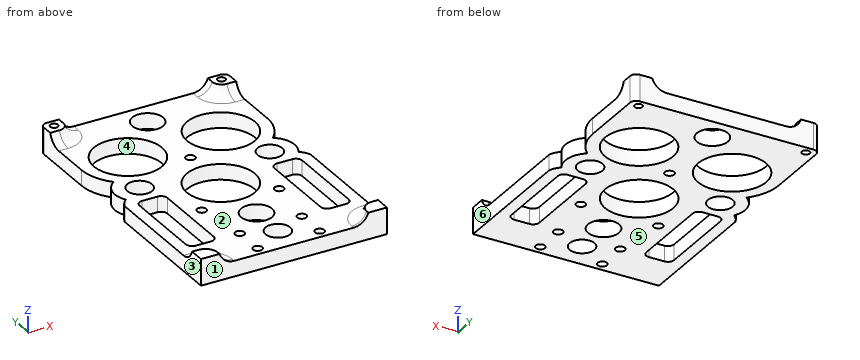
from build123d import *

# Parameters (mm, degrees)
SKETCH1_W            = 60
SKETCH1_H            = 90
BOSS_EXTRUDE1_DEPTH  = 5
SKETCH2_W            = 9
SKETCH2_H            = 30
CUT_EXTRUDE1_DEPTH   = 55.313902456
FILLET1_R            = 2
BOSS_EXTRUDE2_DEPTH  = 3.5
FILLET2_R            = 5
FILLET2_OF_MIRROR1_R = 5
BOSS_EXTRUDE3_DEPTH  = 3.5
SKETCH5_R            = 1.25
CUT_EXTRUDE2_DEPTH   = 55.747146044
FILLET3_R            = 5
FILLET3_OF_MIRROR4_R = 5
FILLET4_R            = 2
SKETCH6_R            = 1.5
CUT_EXTRUDE3_DEPTH   = 55.747146044
SKETCH7_R            = 11
SKETCH7_R_2          = 5
SKETCH7_R_3          = 4
CUT_EXTRUDE4_DEPTH   = 55.313902456


with BuildPart() as part:
    # Sketch1 → Boss-Extrude1 (new body)
    with BuildSketch(Plane.XY):
        Rectangle(SKETCH1_W, SKETCH1_H)
    extrude(amount=BOSS_EXTRUDE1_DEPTH)

    # Sketch2 → Cut-Extrude1 (cut, through all)
    with BuildSketch(Plane(origin=(0, 0, 0), x_dir=(-1, 0, 0), z_dir=(0, 0, -1))):
        with Locations((-21.75, -17)):
            Rectangle(SKETCH2_W, SKETCH2_H)
        with Locations((21.75, -17)):
            Rectangle(SKETCH2_W, SKETCH2_H)
    extrude(amount=-CUT_EXTRUDE1_DEPTH, mode=Mode.SUBTRACT)

    # Fillet1
    fillet1_edges = [part.edges().sort_by_distance(p)[0] for p in [
        (26.25, -32, 2.5),
        (26.25, -2, 2.5),
        (17.25, -2, 2.5),
        (17.25, -32, 2.5),
        (-17.25, -32, 2.5),
        (-17.25, -2, 2.5),
        (-26.25, -2, 2.5),
        (-26.25, -32, 2.5),
    ]]
    fillet(fillet1_edges, radius=FILLET1_R)

    # Sketch3 → Boss-Extrude2 (add)
    with BuildSketch(Plane.XY.offset(5)):
        with BuildLine():
            Line((28, -40), (30, -40))
            Line((30, -40), (30, -45))
            Line((30, -45), (24, -45))
            Line((24, -45), (24, -44))
            ThreePointArc((24, -44), (25.171572875, -41.171572875), (28, -40))
        make_face()
    boss_extrude2 = extrude(amount=BOSS_EXTRUDE2_DEPTH)

    # Fillet2
    # the kernel refuses this fillet: 5 mm, written as the material it adds along each edge
    with BuildSketch(Plane(origin=(28, -40, 5), x_dir=(0, 1, 0), z_dir=(1, 0, 0))) as fillet2_piece_1:
        with BuildLine():
            CenterArc((4.769696007, 5), FILLET2_R, 197.457603124, 72.542396876)
            Line((0, 3.5), (-0.09539392, 3.47))
            ThreePointArc((-0.09539392, 3.47), (-0.1, 1.75), (-0.1, 0))
            Line((-0.1, 0), (0, -0.1))
            Line((0, -0.1), (4.769696007, -0.1))
            Line((4.769696007, -0.1), (4.769696007, 0))
        make_face()
    extrude(amount=2)
    with BuildSketch(Plane(origin=(24, -45, 5), x_dir=(-1, 0, 0), z_dir=(0, 1, 0))) as fillet2_piece_2:
        with BuildLine():
            CenterArc((4.769696007, 5), FILLET2_R, 197.457603124, 72.542396876)
            Line((0, 3.5), (-0.09539392, 3.47))
            ThreePointArc((-0.09539392, 3.47), (-0.1, 1.75), (-0.1, 0))
            Line((-0.1, 0), (0, -0.1))
            Line((0, -0.1), (4.769696007, -0.1))
            Line((4.769696007, -0.1), (4.769696007, 0))
        make_face()
    extrude(amount=1)
    with BuildSketch(Plane(origin=(28, -44, 5), x_dir=(-1, 0, 0), z_dir=(0, -1, 0))) as fillet2_piece_3:
        with BuildLine():
            CenterArc((8.769696007, -5), FILLET2_R, 90, 72.542396876)
            Line((4, -3.5), (3.90460608, -3.47))
            ThreePointArc((3.90460608, -3.47), (3.9, -1.75), (3.9, 0))
            Line((3.9, 0), (4, 0.1))
            Line((4, 0.1), (8.769696007, 0.1))
            Line((8.769696007, 0.1), (8.769696007, 0))
        make_face()
    revolve(axis=Axis((28, -44, 5), (0, 0, -1)), revolution_arc=90)

    # Mirror1: Boss-Extrude2 across plane
    add(boss_extrude2.mirror(Plane(origin=(0, 0, 0), x_dir=(0, 0, 1), z_dir=(1, 0, 0))))

    # Fillet2 of Mirror1
    # the kernel refuses this fillet: 5 mm, written as the material it adds along each edge
    with BuildSketch(Plane(origin=(-28, -40, 5), x_dir=(0, 0, 1), z_dir=(-1, 0, 0))) as fillet2_of_mirror1_piece_1:
        with BuildLine():
            CenterArc((5, 4.769696007), FILLET2_OF_MIRROR1_R, 180, 72.542396876)
            Line((0, 4.769696007), (-0.1, 4.769696007))
            Line((-0.1, 4.769696007), (-0.1, 0))
            Line((-0.1, 0), (0, -0.1))
            ThreePointArc((0, -0.1), (1.75, -0.1), (3.47, -0.09539392))
            Line((3.47, -0.09539392), (3.5, 0))
        make_face()
    extrude(amount=2)
    with BuildSketch(Plane(origin=(-24, -45, 5), x_dir=(0, 0, 1), z_dir=(0, 1, 0))) as fillet2_of_mirror1_piece_2:
        with BuildLine():
            CenterArc((5, 4.769696007), FILLET2_OF_MIRROR1_R, 180, 72.542396876)
            Line((0, 4.769696007), (-0.1, 4.769696007))
            Line((-0.1, 4.769696007), (-0.1, 0))
            Line((-0.1, 0), (0, -0.1))
            ThreePointArc((0, -0.1), (1.75, -0.1), (3.47, -0.09539392))
            Line((3.47, -0.09539392), (3.5, 0))
        make_face()
    extrude(amount=1)
    with BuildSketch(Plane(origin=(-28, -44, 5), x_dir=(1, 0, 0), z_dir=(0, -1, 0))) as fillet2_of_mirror1_piece_3:
        with BuildLine():
            CenterArc((8.769696007, 5), FILLET2_OF_MIRROR1_R, 197.457603124, 72.542396876)
            Line((8.769696007, 0), (8.769696007, -0.1))
            Line((8.769696007, -0.1), (4, -0.1))
            Line((4, -0.1), (3.9, 0))
            ThreePointArc((3.9, 0), (3.9, 1.75), (3.90460608, 3.47))
            Line((3.90460608, 3.47), (4, 3.5))
        make_face()
    revolve(axis=Axis((-28, -44, 5), (0, 0, 1)), revolution_arc=90)

    # Sketch4 → Boss-Extrude3 (add)
    with BuildSketch(Plane.XY.offset(5)):
        with BuildLine():
            Line((24, 45), (24, 42.5))
            ThreePointArc((24, 42.5), (24.878679656, 40.378679656), (27, 39.5))
            Line((27, 39.5), (30, 39.5))
            Line((30, 39.5), (30, 45))
            Line((30, 45), (24, 45))
        make_face()
    boss_extrude3 = extrude(amount=BOSS_EXTRUDE3_DEPTH)

    # Sketch5 → Cut-Extrude2 (cut, through all)
    with BuildSketch(Plane.XY.offset(8.5)):
        with Locations((27, 42.5)):
            Circle(SKETCH5_R)
    cut_extrude2 = extrude(amount=-CUT_EXTRUDE2_DEPTH, mode=Mode.SUBTRACT)

    # Fillet3
    # the kernel refuses this fillet: 5 mm, written as the material it adds along each edge
    with BuildSketch(Plane(origin=(24, 45, 5), x_dir=(-1, 0, 0), z_dir=(0, -1, 0))) as fillet3_piece_1:
        with BuildLine():
            CenterArc((4.769696007, -5), FILLET3_R, 90, 72.542396876)
            Line((0, -3.5), (-0.09539392, -3.47))
            ThreePointArc((-0.09539392, -3.47), (-0.1, -1.75), (-0.1, 0))
            Line((-0.1, 0), (0, 0.1))
            Line((0, 0.1), (4.769696007, 0.1))
            Line((4.769696007, 0.1), (4.769696007, 0))
        make_face()
    extrude(amount=2.5)
    with BuildSketch(Plane(origin=(27, 42.5, 5), x_dir=(-1, 0, 0), z_dir=(0, 1, 0))) as fillet3_piece_2:
        with BuildLine():
            CenterArc((7.769696007, 5), FILLET3_R, 197.457603124, 72.542396876)
            Line((3, 3.5), (2.90460608, 3.47))
            ThreePointArc((2.90460608, 3.47), (2.9, 1.75), (2.9, 0))
            Line((2.9, 0), (3, -0.1))
            Line((3, -0.1), (7.769696007, -0.1))
            Line((7.769696007, -0.1), (7.769696007, 0))
        make_face()
    revolve(axis=Axis((27, 42.5, 5), (0, 0, 1)), revolution_arc=90)
    with BuildSketch(Plane(origin=(27, 39.5, 5), x_dir=(0, -1, 0), z_dir=(1, 0, 0))) as fillet3_piece_3:
        with BuildLine():
            CenterArc((4.769696007, -5), FILLET3_R, 90, 72.542396876)
            Line((0, -3.5), (-0.09539392, -3.47))
            ThreePointArc((-0.09539392, -3.47), (-0.1, -1.75), (-0.1, 0))
            Line((-0.1, 0), (0, 0.1))
            Line((0, 0.1), (4.769696007, 0.1))
            Line((4.769696007, 0.1), (4.769696007, 0))
        make_face()
    extrude(amount=3)

    # Mirror4: Boss-Extrude3, Cut-Extrude2 across plane
    add(boss_extrude3.mirror(Plane(origin=(0, 0, 0), x_dir=(0, 0, 1), z_dir=(1, 0, 0))))
    add(cut_extrude2.mirror(Plane(origin=(0, 0, 0), x_dir=(0, 0, 1), z_dir=(1, 0, 0))), mode=Mode.SUBTRACT)

    # Fillet3 of Mirror4
    # the kernel refuses this fillet: 5 mm, written as the material it adds along each edge
    with BuildSketch(Plane(origin=(-24, 45, 5), x_dir=(1, 0, 0), z_dir=(0, -1, 0))) as fillet3_of_mirror4_piece_1:
        with BuildLine():
            CenterArc((4.769696007, 5), FILLET3_OF_MIRROR4_R, 197.457603124, 72.542396876)
            Line((0, 3.5), (-0.09539392, 3.47))
            ThreePointArc((-0.09539392, 3.47), (-0.1, 1.75), (-0.1, 0))
            Line((-0.1, 0), (0, -0.1))
            Line((0, -0.1), (4.769696007, -0.1))
            Line((4.769696007, -0.1), (4.769696007, 0))
        make_face()
    extrude(amount=2.5)
    with BuildSketch(Plane(origin=(-27, 42.5, 5), x_dir=(1, 0, 0), z_dir=(0, 1, 0))) as fillet3_of_mirror4_piece_2:
        with BuildLine():
            CenterArc((7.769696007, -5), FILLET3_OF_MIRROR4_R, 90, 72.542396876)
            Line((3, -3.5), (2.90460608, -3.47))
            ThreePointArc((2.90460608, -3.47), (2.9, -1.75), (2.9, 0))
            Line((2.9, 0), (3, 0.1))
            Line((3, 0.1), (7.769696007, 0.1))
            Line((7.769696007, 0.1), (7.769696007, 0))
        make_face()
    revolve(axis=Axis((-27, 42.5, 5), (0, 0, -1)), revolution_arc=90)
    with BuildSketch(Plane(origin=(-27, 39.5, 5), x_dir=(0, -1, 0), z_dir=(-1, 0, 0))) as fillet3_of_mirror4_piece_3:
        with BuildLine():
            CenterArc((4.769696007, 5), FILLET3_OF_MIRROR4_R, 197.457603124, 72.542396876)
            Line((0, 3.5), (-0.09539392, 3.47))
            ThreePointArc((-0.09539392, 3.47), (-0.1, 1.75), (-0.1, 0))
            Line((-0.1, 0), (0, -0.1))
            Line((0, -0.1), (4.769696007, -0.1))
            Line((4.769696007, -0.1), (4.769696007, 0))
        make_face()
    extrude(amount=3)

    # Fillet4
    fillet4_edges = [part.edges().sort_by_distance(p)[0] for p in [
        (-30, 45, 4.25),
        (30, 45, 4.25),
    ]]
    fillet(fillet4_edges, radius=FILLET4_R)

    # Sketch6 → Cut-Extrude3 (cut, through all)
    with BuildSketch(Plane(origin=(0, 0, 0), x_dir=(-1, 0, 0), z_dir=(0, 0, -1))):
        with Locations((-10, -32)):
            Circle(SKETCH6_R)
        with Locations((-10, -42)):
            Circle(SKETCH6_R)
        with Locations((10, -42)):
            Circle(SKETCH6_R)
        with Locations((10, -32)):
            Circle(SKETCH6_R)
        with Locations((0, 13)):
            Circle(SKETCH6_R)
        with Locations((12.5, -15)):
            Circle(SKETCH6_R)
        with Locations((-12.5, -15)):
            Circle(SKETCH6_R)
    extrude(amount=-CUT_EXTRUDE3_DEPTH, mode=Mode.SUBTRACT)

    # Sketch7 → Cut-Extrude4 (cut, through all)
    with BuildSketch(Plane.XY.offset(5)):
        with Locations((-15, 22)):
            Circle(SKETCH7_R)
        with Locations((15, 22)):
            Circle(SKETCH7_R)
        with Locations((0, -4)):
            Circle(SKETCH7_R)
        with Locations((0, -24)):
            Circle(SKETCH7_R_2)
        with Locations((0, -36)):
            Circle(SKETCH7_R_3)
        with Locations((0, 37)):
            Circle(SKETCH7_R_2)
        with Locations((-21, 5)):
            Circle(SKETCH7_R_3)
        with Locations((21, 5)):
            Circle(SKETCH7_R_3)
        with BuildLine():
            Line((30, 22), (30, 5))
            Line((30, 5), (30, -2.28608635))
            ThreePointArc((30, -2.28608635), (29.162980054, -0.555783544), (27.82175868, 0.821051746))
            ThreePointArc((27.82175868, 0.821051746), (28.844928487, 6.567513007), (25.692059794, 11.479550516))
            ThreePointArc((25.692059794, 11.479550516), (28.881298515, 16.315850852), (30, 22))
        make_face()
        with BuildLine():
            Line((-30, 5), (-30, -2.28608635))
            ThreePointArc((-30, -2.28608635), (-29.162980054, -0.555783544), (-27.82175868, 0.821051746))
            ThreePointArc((-27.82175868, 0.821051746), (-28.844928487, 6.567513007), (-25.692059794, 11.479550516))
            ThreePointArc((-25.692059794, 11.479550516), (-28.881298515, 16.315850852), (-30, 22))
            Line((-30, 22), (-30, 5))
        make_face()
    extrude(amount=-CUT_EXTRUDE4_DEPTH, mode=Mode.SUBTRACT)


solid = part.part
The listing builds one solid part. Answer for the finished solid, in the listing's coordinates (mm). Face numbers are marked on the shaded views. A direction names the side the tool comes from. Coordinates: 2 decimals unless noted, no trailing zeros. Order: outer loops, then holes, each group sorted by start corner. A loop starts at its lowest first (then second) coordinate and runs counter-clockwise, first axis right, second up. Notation, with made-up numbers: M 53.5,29 L 71.5,29 A15 cw 71.5,41 Z; hole C 22,-19 d7. An arc over 180 degrees is marked long. Use CSV: the item, a comma, the result in double quotes.
Q1. Section D-D (x = 10) is taken. Determine the outline of the cut face in (y, z).
Here are the results:
outline,"M -45,0 L -43.5,0 L -43.5,5 L -45,5 Z; M -40.5,0 L -33.5,0 L -33.5,5 L -40.5,5 Z; M -30.5,0 L -8.58,0 L -8.58,5 L -30.5,5 Z; M 0.58,0 L 12.2,0 L 12.2,5 L 0.58,5 Z; M 31.8,0 L 45,0 L 45,5 L 31.8,5 Z"
Q2. Determine the mould class of the marked faces 3, 4, 5 and 6 for opening direction X: pulls with the +X half, pulls with the -X half, needs draft (parallel to the pull), parting line crosses it, or undercut.
Here are the results:
face 3,"pulls with the -X half"
face 4,"undercut"
face 5,"needs draft"
face 6,"pulls with the +X half"
Q3. A tool of negligible diameter and unlimited length cuts with its end or side. For the marked faces 1 and 2, from which of +Z, -Z, +X, -X, +Y, -Y can it reach the whole face along a straight path? Write none if from no direction.
Here are the results:
face 1,"+Z, -Z, +X, -X, -Y"
face 2,"+Z"
Q4. Straight lines are drawn through the part: L1, parallel to Y at x = 0, z = 1.1; L2, parallel to Y at x = 7.5, z = 1.5; L3, parallel to X at y = 25.5, z = 1.5. For each, find the intervals that lie inside material, in ascending order.
Here are the results:
L1,"-45 to -40, -32 to -29, -19 to -15, 7 to 11.5, 14.5 to 32, 42 to 45"
L2,"-45 to -12.05, 4.05 to 13.95, 30.05 to 45"
L3,"-30 to -25.43, -4.57 to 4.57, 25.43 to 30"
Q5. Section B-B (z = 6.5) is taken. Determine the outline of the cut face in (x, y).
Here are the results:
outline,"M -30,-45 L -22.8,-45 L -22.8,-44 A5.2 ccw -28,-38.8 L -30,-38.8 Z; M -30,38.3 L -27,38.3 A4.2 ccw -22.8,42.5 L -22.8,45 L -28,45 A2 ccw -30,43 Z; M 22.8,-45 L 30,-45 L 30,-38.8 L 28,-38.8 A5.2 ccw 22.8,-44 Z; M 22.8,42.5 A4.2 ccw 27,38.3 L 30,38.3 L 30,43 A2 ccw 28,45 L 22.8,45 Z; hole C -27,42.5 d2.5; hole C 27,42.5 d2.5"
Q6. Section A-A (x = -15) is taken. Determine the outline of the cut face in (y, z), then the cut area to 3 significant figures.
Here are the results:
outline,"M -45,0 L 11,0 L 11,5 L -45,5 Z; M 33,0 L 45,0 L 45,5 L 33,5 Z"
area,"340 mm2"
Q7. Section C-C (y = 20.5) is taken. Determine the outline of the cut face in (x, z).
Here are the results:
outline,"M -29.92,0 L -25.9,0 L -25.9,5 L -29.92,5 Z; M -4.1,0 L 4.1,0 L 4.1,5 L -4.1,5 Z; M 25.9,0 L 29.92,0 L 29.92,5 L 25.9,5 Z"
Q8. Given pin 1 Ø10.5 at (x, y) = (21, 5) entering from -Z; pin 2 Ø11.5 at (x, y) = (0, -24) entering from +Z, each flat-ended and moving along its own axis, determine where each tip first touches the part or whether it passes through.
Here are the results:
pin 1,"z = 0"
pin 2,"z = 5"
